Verification items for the finished model (mm, model axes). A direction names the side the tool comes from. Round coordinates to 2 decimals unless told otherwise and drop trailing zeros. One line per item, written item: value. Start each with the question number.
from build123d import *

# Parameters (mm, degrees)
SKETCH_3_R      = 4
SKETCH_3_R_2    = 3
SKETCH_3_R_3    = 1.5
SKETCH_3_R_4    = 1.500000004
SKETCH_3_R_5    = 1.499999999
SKETCH_3_W      = 23.6
SKETCH_3_H      = 12.6
SKETCH_3_W_2    = 4
SKETCH_3_H_2    = 2.8
EXTRUDE_3_DEPTH = 2.8


with BuildPart() as part:
    # Эскиз3 → Бобышка-Вытянуть3 (new body)
    with BuildSketch(Plane.XY):
        with BuildLine():
            Line((200, 0.21), (200, -0.21))
            add(Edge.make_bspline(
                [(173.839461144, -3.040801203), (175.943333039, -2.830170954), (179.564023078, -2.461029339), (184.58704572, -1.932479181), (188.771568451, -1.480695182), (192.530784687, -1.065063842), (195.747560944, -0.701689979), (198.179524953, -0.422303954), (199.520051416, -0.265971644), (200, -0.21)],
                knots=[0.870307302, 0.870307302, 0.870307302, 0.870307302, 0.901571134, 0.924121062, 0.944988816, 0.963803939, 0.980044339, 0.992855276, 1, 1, 1, 1], degree=3))
            Line((173.839461144, -3.040801203), (162.170244806, -4.170244806))
            add(Edge.make_bspline(
                [(100.4, -8.802264), (100.782530515, -8.78200637), (103.102887785, -8.657921344), (107.374551667, -8.416266925), (113.223109349, -8.057497647), (119.097620698, -7.671146294), (124.98256269, -7.259840679), (130.861479372, -6.826169971), (136.716836604, -6.372892076), (142.52985565, -5.902766003), (148.280267017, -5.418602057), (153.94609331, -4.923426646), (158.566687276, -4.50520567), (161.295968592, -4.251994411), (162.170244806, -4.170244806)],
                knots=[0.507199784, 0.507199784, 0.507199784, 0.507199784, 0.512863887, 0.541558094, 0.570462313, 0.599504248, 0.628607349, 0.657690446, 0.686667237, 0.715444849, 0.743923546, 0.77199483, 0.799540253, 0.812523886, 0.812523886, 0.812523886, 0.812523886], degree=3))
            Line((100.4, -8.802264), (100.4, -5.802264))
            Line((100.4, -5.802264), (97.6, -5.802264))
            Line((97.6, -5.802264), (97.6, -8.946938935))
            add(Edge.make_bspline(
                [(96.16294038, -9.018329177), (96.641976589, -8.994862294), (97.120996479, -8.971063118), (97.6, -8.946938935)],
                knots=[0.486289284, 0.486289284, 0.486289284, 0.486289284, 0.493380908, 0.493380908, 0.493380908, 0.493380908], degree=3))
            ThreePointArc((96.16294038, -9.018329177), (91.867526446, -13.724080291), (87.17182932, -9.417677743))
            add(Edge.make_bspline(
                [(48.849842288, -9.876307099), (50.29548458, -9.910701869), (53.368870018, -9.967597185), (58.119580476, -10.007674079), (63.1472323, -10.001179647), (68.312112853, -9.948180779), (73.603706203, -9.849984193), (79.011121779, -9.708185508), (83.546665754, -9.557168434), (86.278412172, -9.453068368), (87.17182932, -9.417677743)],
                knots=[0.253007448, 0.253007448, 0.253007448, 0.253007448, 0.274388983, 0.298458209, 0.323253842, 0.348727971, 0.374830387, 0.40150919, 0.428710016, 0.441930624, 0.441930624, 0.441930624, 0.441930624], degree=3))
            ThreePointArc((48.849842288, -9.876307099), (44.191437181, -14.24080929), (39.855729482, -9.55559251))
            add(Edge.make_bspline(
                [(15.984525285, -7.176038428), (16.462030484, -7.259158951), (17.98454817, -7.513637269), (20.631718929, -7.904294519), (23.999672572, -8.325205071), (27.586779878, -8.701741845), (31.384869898, -9.032475932), (35.385580654, -9.316092874), (38.232256125, -9.476007566), (39.743803487, -9.550160154), (39.855729482, -9.55559251)],
                knots=[0.090340762, 0.090340762, 0.090340762, 0.090340762, 0.097507218, 0.113164082, 0.12990269, 0.147690304, 0.166492185, 0.186271967, 0.206991861, 0.208648761, 0.208648761, 0.208648761, 0.208648761], degree=3))
            ThreePointArc((15.984525285, -7.176038428), (10.553276044, -10.683492951), (7.222061882, -5.142399398))
            add(Edge.make_bspline(
                [(0, 0), (0.032444913, -0.278495812), (0.100633198, -0.863800259), (0.62379252, -1.678905598), (1.407454519, -2.445359097), (2.482159911, -3.178007514), (3.831515726, -3.881540279), (5.438246861, -4.54900077), (6.605008441, -4.947778836), (7.222061882, -5.142399398)],
                knots=[0, 0, 0, 0, 0.004099011, 0.008614742, 0.013934855, 0.020277775, 0.027752981, 0.036410215, 0.045976094, 0.045976094, 0.045976094, 0.045976094], degree=3))
            add(Edge.make_bspline(
                [(19.284694791, 7.702161614), (18.661991317, 7.611303464), (17.067549655, 7.367338744), (14.58489291, 6.936612431), (11.921305119, 6.393879384), (9.507426038, 5.81478546), (7.350195056, 5.201638101), (5.45639967, 4.556541724), (3.831515725, 3.88154028), (2.48215991, 3.178007515), (1.407454518, 2.445359098), (0.62379252, 1.678905598), (0.100633198, 0.863800259), (0.032444913, 0.278495812), (0, 0)],
                knots=[0.893188074, 0.893188074, 0.893188074, 0.893188074, 0.902492782, 0.917037139, 0.930441054, 0.942679762, 0.953733567, 0.963589785, 0.972247019, 0.979722225, 0.986065145, 0.991385258, 0.995900989, 1, 1, 1, 1], degree=3))
            ThreePointArc((19.284694791, 7.702161614), (23.222530105, 12.753724018), (28.222638882, 8.75075738))
            add(Edge.make_bspline(
                [(63.6, 9.990751447), (63.433767139, 9.991846739), (61.590618822, 10.003190391), (58.119580476, 10.007674079), (53.23934089, 9.96650448), (48.51637403, 9.877065972), (43.960263435, 9.738807032), (39.580313293, 9.551735955), (35.385580654, 9.316092874), (31.619699098, 9.049123359), (29.254379223, 8.84661187), (28.222638882, 8.75075738)],
                knots=[0.674288155, 0.674288155, 0.674288155, 0.674288155, 0.676746158, 0.701541791, 0.725611017, 0.748907835, 0.771387785, 0.793008139, 0.813728033, 0.833507815, 0.84882888, 0.84882888, 0.84882888, 0.84882888], degree=3))
            Line((63.6, 9.990751447), (63.6, 6.965595937))
            Line((63.6, 6.965595937), (66.4, 6.965595937))
            Line((66.4, 6.965595937), (66.4, 9.965595937))
            add(Edge.make_bspline(
                [(95.498574643, 9.050660645), (93.699350388, 9.137637837), (90.030763168, 9.305301287), (84.52309051, 9.524657051), (79.011121778, 9.708185508), (73.603706202, 9.849984193), (69.41154014, 9.927778606), (67.023185068, 9.958531818), (66.4, 9.965595937)],
                knots=[0.516989075, 0.516989075, 0.516989075, 0.516989075, 0.543623846, 0.571289984, 0.59849081, 0.625169613, 0.651272029, 0.660487149, 0.660487149, 0.660487149, 0.660487149], degree=3))
            ThreePointArc((95.498574643, 9.050660645), (100.228464185, 13.308356698), (104.486160238, 8.578467155))
            add(Edge.make_bspline(
                [(124, 7.326294797), (122.364596134, 7.442700413), (118.769611386, 7.692718614), (113.223109349, 8.057497647), (108.353742435, 8.356200224), (105.444206381, 8.524292737), (104.486160238, 8.578467155)],
                knots=[0.376253135, 0.376253135, 0.376253135, 0.376253135, 0.400495752, 0.429537687, 0.458441906, 0.47263041, 0.47263041, 0.47263041, 0.47263041], degree=3))
            Line((124, 7.326294797), (124, 4.124412105))
            Line((124, 4.124412105), (126.8, 4.124412105))
            Line((126.8, 4.124412105), (126.8, 7.124412105))
            add(Edge.make_bspline(
                [(200, 0.21), (199.520051416, 0.265971644), (198.179524953, 0.422303954), (195.747560944, 0.701689979), (192.530784687, 1.065063842), (188.771568451, 1.480695182), (184.58704572, 1.932479181), (180.05616868, 2.409243063), (175.238405485, 2.90257428), (168.371896377, 3.585728287), (161.260104983, 4.261418012), (153.94609331, 4.923426646), (148.280267017, 5.418602057), (142.52985565, 5.902766003), (136.716836604, 6.372892076), (131.466708661, 6.779317653), (128.156255998, 7.025385403), (126.8, 7.124412105)],
                knots=[0, 0, 0, 0, 0.007144724, 0.019955661, 0.036196061, 0.055011184, 0.075878938, 0.098428866, 0.122375554, 0.147487885, 0.200459747, 0.22800517, 0.256076454, 0.284555151, 0.313332763, 0.342309554, 0.362416837, 0.362416837, 0.362416837, 0.362416837], degree=3))
        make_face()
        with Locations((109, 0)):
            Circle(SKETCH_3_R, mode=Mode.SUBTRACT)
        with Locations((55, 0)):
            Circle(SKETCH_3_R, mode=Mode.SUBTRACT)
        with Locations((150, 0)):
            Circle(SKETCH_3_R_2, mode=Mode.SUBTRACT)
        with Locations((68.565, 0)):
            Circle(SKETCH_3_R_3, mode=Mode.SUBTRACT)
        with Locations((95.435, 0)):
            Circle(SKETCH_3_R_3, mode=Mode.SUBTRACT)
        with Locations((23.746872016, 10.284376689)):
            Circle(SKETCH_3_R_4, mode=Mode.SUBTRACT)
        with Locations((11.570620364, -8.299999991)):
            Circle(SKETCH_3_R_5, mode=Mode.SUBTRACT)
        with Locations((44.351797521, -11.743667469)):
            Circle(SKETCH_3_R_5, mode=Mode.SUBTRACT)
        with Locations((91.667851618, -11.228512478)):
            Circle(SKETCH_3_R_3, mode=Mode.SUBTRACT)
        with Locations((99.99236744, 10.8145639)):
            Circle(SKETCH_3_R_3, mode=Mode.SUBTRACT)
        with BuildLine():
            Line((19.3, 5), (42.3, 5))
            ThreePointArc((42.3, 5), (47.3, 0), (42.3, -5))
            Line((42.3, -5), (19.3, -5))
            ThreePointArc((19.3, -5), (14.3, 0), (19.3, 5))
        make_face(mode=Mode.SUBTRACT)
        with BuildLine():
            Line((119.34345336, 1.992816182), (134.326801485, 2.699412943))
            ThreePointArc((134.326801485, 2.699412943), (137.987788625, -0.631829042), (134.65654664, -4.292816182))
            Line((134.65654664, -4.292816182), (119.673198515, -4.999412943))
            ThreePointArc((119.673198515, -4.999412943), (116.012211375, -1.668170958), (119.34345336, 1.992816182))
        make_face(mode=Mode.SUBTRACT)
        with Locations((82, 0)):
            Rectangle(SKETCH_3_W, SKETCH_3_H, mode=Mode.SUBTRACT)
        with Locations((164, 0)):
            Rectangle(SKETCH_3_W_2, SKETCH_3_H_2, mode=Mode.SUBTRACT)
    extrude(amount=EXTRUDE_3_DEPTH)


solid = part.part
1) Thickness scan on line 1 (Y direction, x = 55, z = 1.3); line 2 (Y direction, x = 62, z = 1.8); line 3 (Y direction, x = 150, z = 1.5). Record the ranges inside material, lowest first.
2) Access from +Z, -Z, +X, -X, +Y, -Y to the whole of each face (thin tool, end or side, straight path). Record for faces 3 (the cylindrical face through (47.3, 0.1, 1.4)), 4 (the flat face through (101, 0, 0)).
3) Gauge pin test, flat ends, axial feed: pin 1 Ø1.4 at (y, z) = (2, 1) entering from -X; pin 2 Ø0.8 at (x, z) = (30.5, 1.5) entering from +Y; pin 3 Ø1 at (y, z) = (-9.5, 2.5) entering from -X. Record the tip position at first contact, or that the pin passes through.
4) Mould release check, pull along Y, two halves, no side actions. Record for faces 1 (the flat face through (101, 0, 2.8)), 2 (the cylindrical face through (137.983, -0.555, 1.38)): pulls with the +Y half, pulls with the -Y half, needs draft (parallel to the pull), parting line crosses it, or undercut.
5) Cross-section at A-A (z = 0.45). State how many separate pieces and enclosed holes the cut face has, then the cut area to 3 significant figures.
Results below:
1. line 1: y = -9.98 to -4, 4 to 9.98
1. line 2: y = -10 to 10
1. line 3: y = -5.27 to -3, 3 to 5.27
2. face 3: +Z, -Z
2. face 4: -Z, +X, -X, +Y, -Y
3. pin 1: stops at x = 0.39
3. pin 2: stops at y = 8.98
3. pin 3: stops at x = 7.97
4. face 1: needs draft
4. face 2: undercut
5. separate pieces: 1
5. enclosed holes: 14
5. area: 1,940 mm²
